Could you check a few things on this drawing? It's one solid part, dimensions in mm from its lowest x, y, z. A direction names the side the tool comes from. Give positions to 0.01 mm unless a question says otherwise; leave off trailing zeros. Order: outer loops, then holes, each group sorted by start corner. A loop starts at its lowest first (then second) coordinate and runs counter-clockwise, first axis right, second up. Notation, with made-up numbers: (-6, 55.5) - (-2, 55.5) arc R23 cw to (-2, 88.5) - close; hole circle Ø1 at (-25.75, 61.25). An arc over 180 degrees is marked (long way). Return JSON: item names as keys, results as strings.
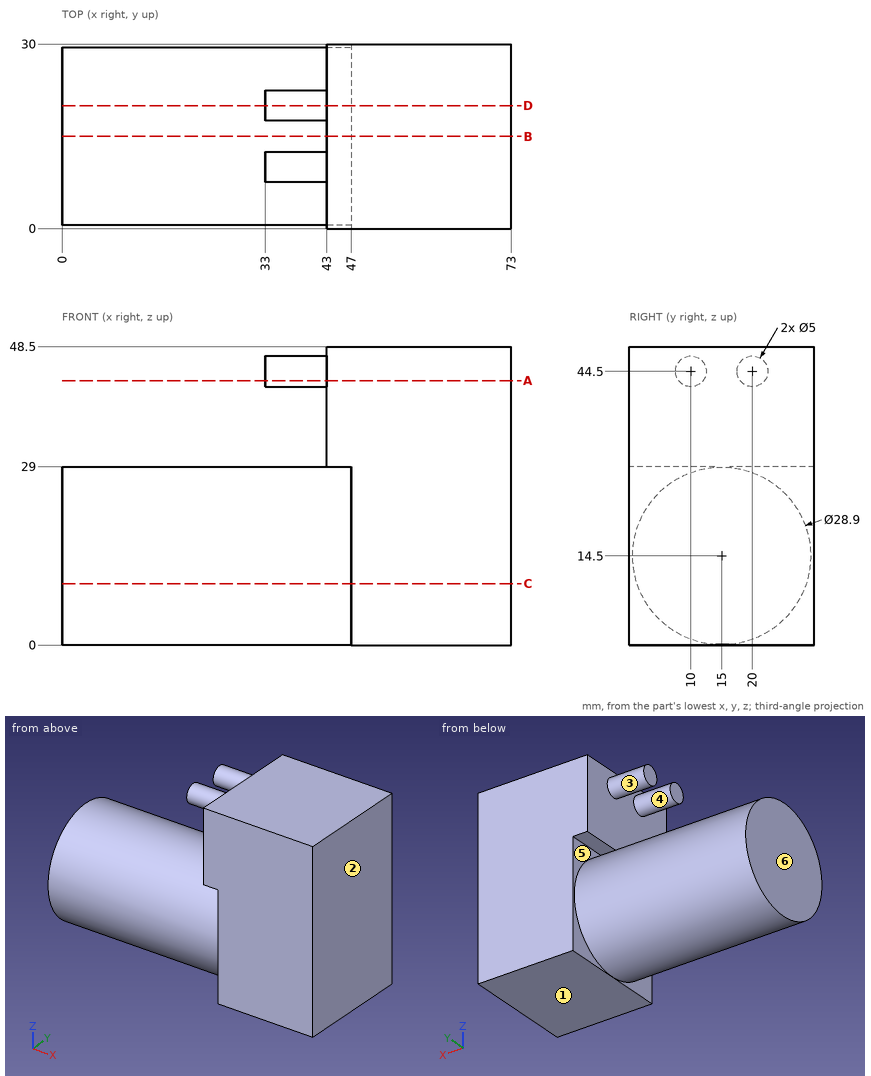
1. Suppose I cut it at C-C (z = 10). List the corners of the cut face in (x, y) for me, plus the area to 3 significant figures.
Checks:
{"outline": "(0, 1.27) - (47, 1.27) - (47, 0) - (73, 0) - (73, 30) - (47, 30) - (47, 28.73) - (0, 28.73) - close", "area": "2,070 mm^2"}
2. If I drill on L1, parallel to X at y = 8.75, z = 33.5; L2, parallel to X at y = 10.75, z = 43; L3, parallel to Y at x = 11.5, z = 25, over which ranges is the centre line in solid material (lowest first)? Write a range as [from, to].
Checks:
{"L1": "[43, 73]", "L2": "[33, 73]", "L3": "[5.07, 24.93]"}
3. On a 3-axis mill with a long thin cutter (end or side, diameter ignored), from which of +Z, -Z, +X, -X, +Y, -Y can I reach the whole of each face in a straight line? I mean the marked faces 5 and 6. Say none if no direction works.
Checks:
{"face 5": "-X", "face 6": "+Z, -Z, -X, +Y, -Y"}
4. For pin 1 Ø4 at (x, y) = (16, 22) entering from +Z; pin 2 Ø2 at (x, z) = (34, 13.5) entering from +Y; pin 3 Ø10 at (x, y) = (27.5, 9) entering from +Z, each with a flat end and sliding along its axis, tell me the tip position at first contact or that it passes through.
Checks:
{"pin 1": "z = 28.06", "pin 2": "y = 29.45", "pin 3": "z = 28.92"}
5. Suppose I cut it at D-D (y = 20). List the corners of the cut face in (x, z) for me, plus the area to 3 significant figures.
Checks:
{"outline": "(0, 0.94) - (47, 0.94) - (47, 0) - (73, 0) - (73, 48.5) - (43, 48.5) - (43, 47) - (33, 47) - (33, 42) - (43, 42) - (43, 29) - (47, 29) - (47, 28.06) - (0, 28.06) - close", "area": "2,660 mm^2"}
6. Suppose I cut it at B-B (y = 15). List the corners of the cut face in (x, z) for me, plus the area to 3 significant figures.
Checks:
{"outline": "(0, 0.05) - (47, 0.05) - (47, 0) - (73, 0) - (73, 48.5) - (43, 48.5) - (43, 29) - (47, 29) - (47, 28.95) - (0, 28.95) - close", "area": "2,700 mm^2"}
7. Thinking about a two-plate mould opening in Z: for the marked faces 1, 2, 3 and 4, which applies, +Z half, -Z half, draft (parallel to the pull), parting line (faces both ways), or undercut?
Checks:
{"face 1": "-Z half", "face 2": "draft", "face 3": "undercut", "face 4": "undercut"}
8. Suppose I cut it at A-A (z = 43). List the corners of the cut face in (x, y) for me.
Checks:
{"outline": "(33, 8) - (43, 8) - (43, 0) - (73, 0) - (73, 30) - (43, 30) - (43, 22) - (33, 22) - (33, 18) - (43, 18) - (43, 12) - (33, 12) - close"}
